```python
from build123d import *

# Parameters (mm, degrees)
BOSS_EXTRUDE1_DEPTH         = 50.8
SKETCH2_R                   = 12.7
CUT_EXTRUDE1_DEPTH          = 86.09
SKETCH3_R                   = 12.7
BOSS_EXTRUDE2_DEPTH         = 6.35
SKETCH4_R                   = 19.05
BOSS_EXTRUDE3_DEPTH         = 1.27
CUT_EXTRUDE2_REACH          = 150.59
SKETCH5_R                   = 6.35
SKETCH6_R                   = 12.7
BOSS_EXTRUDE4_DEPTH         = 3.81
SKETCH7_R                   = 19.05
BOSS_EXTRUDE5_DEPTH         = 1.27
F_1_16_0_5_DIAMETER_HOLE1_D = 12.7


with BuildPart() as part:
    # Sketch1 → Boss-Extrude1 (new body)
    with BuildSketch(Plane.XY):
        with BuildLine():
            Line((42.545, 113.03), (42.545, -25.4))
            Line((42.545, -25.4), (41.275, -25.4))
            Line((41.275, -25.4), (41.275, 111.76))
            ThreePointArc((41.275, 111.76), (40.531051224, 113.556051224), (38.735, 114.3))
            Line((38.735, 114.3), (-38.735, 114.3))
            ThreePointArc((-38.735, 114.3), (-40.531051224, 113.556051224), (-41.275, 111.76))
            Line((-41.275, 111.76), (-41.275, -25.4))
            Line((-41.275, -25.4), (-42.545, -25.4))
            Line((-42.545, -25.4), (-42.545, 113.03))
            ThreePointArc((-42.545, 113.03), (-41.801051224, 114.826051224), (-40.005, 115.57))
            Line((-40.005, 115.57), (40.005, 115.57))
            ThreePointArc((40.005, 115.57), (41.801051224, 114.826051224), (42.545, 113.03))
        make_face()
    extrude(amount=BOSS_EXTRUDE1_DEPTH)

    # Sketch2 → Cut-Extrude1 (cut, through all)
    with BuildSketch(Plane.ZY.offset(42.545)):
        with Locations((25.4, 0)):
            Circle(SKETCH2_R)
    extrude(amount=-CUT_EXTRUDE1_DEPTH, mode=Mode.SUBTRACT)

    # Sketch3 → Boss-Extrude2 (add)
    with BuildSketch(Plane(origin=(0, 115.57, 0), x_dir=(1, 0, 0), z_dir=(0, 1, 0))):
        with Locations((0, -25.4)):
            Circle(SKETCH3_R)
    extrude(amount=BOSS_EXTRUDE2_DEPTH)

    # Sketch4 → Boss-Extrude3 (add)
    with BuildSketch(Plane(origin=(0, 121.92, 0), x_dir=(1, 0, 0), z_dir=(0, 1, 0))):
        with Locations((0, -25.4)):
            Circle(SKETCH4_R)
    extrude(amount=BOSS_EXTRUDE3_DEPTH)

    # Sketch5 → Cut-Extrude2 (cut, up to next)
    with BuildSketch(Plane(origin=(0, 123.19, 0), x_dir=(1, 0, 0), z_dir=(0, 1, 0)), mode=Mode.PRIVATE) as cut_extrude2_sk1:
        with Locations((0, -25.4)):
            Circle(SKETCH5_R)
    cut_extrude2_tool1 = extrude(cut_extrude2_sk1.sketch, amount=-CUT_EXTRUDE2_REACH, mode=Mode.PRIVATE) & part.part
    add(cut_extrude2_tool1.solids().sort_by_distance((0, 123.19, 25.4))[0], mode=Mode.SUBTRACT)

    # Sketch6 → Boss-Extrude4 (add)
    with BuildSketch(Plane(origin=(0, 123.19, 0), x_dir=(1, 0, 0), z_dir=(0, 1, 0))):
        with Locations((0, -25.4)):
            Circle(SKETCH6_R)
    extrude(amount=BOSS_EXTRUDE4_DEPTH)

    # Sketch7 → Boss-Extrude5 (add)
    with BuildSketch(Plane(origin=(0, 127, 0), x_dir=(1, 0, 0), z_dir=(0, 1, 0))):
        with Locations((0, -25.4)):
            Circle(SKETCH7_R)
    extrude(amount=BOSS_EXTRUDE5_DEPTH)

    # 1/16 (0.5) Diameter Hole1 (through all)
    with Locations(Plane(origin=(0, 128.27, 0), x_dir=(1, 0, 0), z_dir=(0, 1, 0))):
        with Locations((0, -25.4)):
            Hole(F_1_16_0_5_DIAMETER_HOLE1_D / 2)


solid = part.part
```
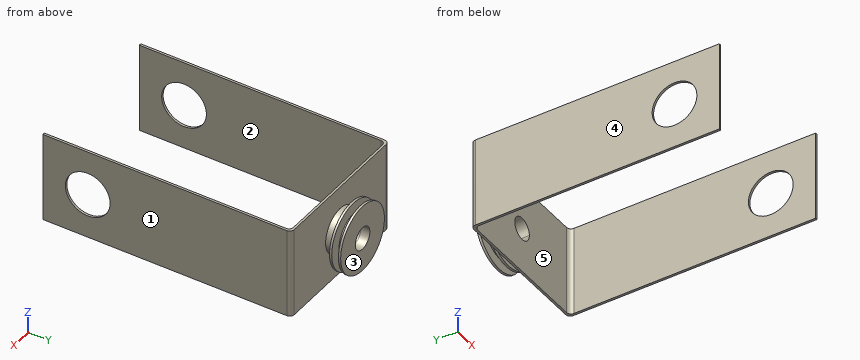
Source: CAD feature listing. Evaluate the final solid. Frame: model axes, mm. Face numbers are marked on the shaded views. A direction names the side the tool comes from. Round coordinates to 2 decimals unless told otherwise and drop trailing zeros. Loops run counter-clockwise (first coordinate to the right, second up) from the corner with the lowest first, then second, coordinate; pieces in that order, holes last. Notation, with made-up numbers: M 43.5,85 L 61.5,85 A25 cw 61.5,97 Z; hole C 62.5,11.5 d3. An arc over 180 degrees is marked long. Put each result on its own line as item: value.
(1) First-contact query: pin 1 (8 mm diameter, centred on x = 33.5, z = 38.5, fed in from -Y); pin 2 (23 mm diameter, centred on y = 0, z = 25.4, fed in from +X). Flat tips, straight axial feed; report the tip coordinate or a pass-through.
Solutions:
pin 1: y = 114.3
pin 2: through
(2) Section B-B, the plane x = 0. Return loops of the section in (y, z).
Solutions:
outline: M 114.3,0 L 115.57,0 L 115.57,12.7 L 121.92,12.7 L 121.92,6.35 L 123.19,6.35 L 123.19,12.7 L 127,12.7 L 127,6.35 L 128.27,6.35 L 128.27,19.05 L 114.3,19.05 Z; M 114.3,31.75 L 128.27,31.75 L 128.27,44.45 L 127,44.45 L 127,38.1 L 123.19,38.1 L 123.19,44.45 L 121.92,44.45 L 121.92,38.1 L 115.57,38.1 L 115.57,50.8 L 114.3,50.8 Z
(3) Section D-D, the plane z = 15. State how many separate pieces and enclosed holes the cut face has, and give its area (3 significant figures).
Solutions:
separate pieces: 3
enclosed holes: 0
area: 655 mm²
(4) Pull-direction query (X, two-part tool) for the marked faces 3, 4 and 5; classes: released by +X, released by -X, zero draft, split by the parting line, or undercut.
Solutions:
face 3: zero draft
face 4: released by -X
face 5: undercut
(5) Section A-A, the plane y = 76. Return loops of the section in (x, z) (3 decimals).
Solutions:
outline: M -42.545,0 L -41.275,0 L -41.275,50.8 L -42.545,50.8 Z; M 41.275,0 L 42.545,0 L 42.545,50.8 L 41.275,50.8 Z
(6) Section C-C, the plane y = 0. Return loops of the section in (x, z) (3 decimals), and give its area (3 significant figures).
Solutions:
outline: M -42.545,0 L -41.275,0 L -41.275,12.7 L -42.545,12.7 Z; M -42.545,38.1 L -41.275,38.1 L -41.275,50.8 L -42.545,50.8 Z; M 41.275,0 L 42.545,0 L 42.545,12.7 L 41.275,12.7 Z; M 41.275,38.1 L 42.545,38.1 L 42.545,50.8 L 41.275,50.8 Z
area: 64.5 mm²
(7) Ray query, line 1 (Z direction, x = 0, y = 126.6); line 2 (X direction, y = 84.5, z = 24) (3 decimals); line 3 (Y direction, x = -31, z = 13.5). Return the intervals inside material, ascending. Write a range as [from, to].
Solutions:
line 1: [12.7, 19.05], [31.75, 38.1]
line 2: [-42.545, -41.275], [41.275, 42.545]
line 3: [114.3, 115.57]
(8) Access query for the marked faces 1 and 2. Directions: +Z, -Z, +X, -X, +Y, -Y. A direction counts if a zero-diameter tool reaches every point of the face in a straight line with its end or side. Return the directions, or none.
Solutions:
face 1: +Z, -Z, +X, +Y, -Y
face 2: +Z, -Z, -Y
